Source: CAD feature listing. Evaluate the final solid. Frame: model axes, mm. A direction names the side the tool comes from. Coordinates: 2 decimals unless noted, no trailing zeros. Order: outer loops, then holes, each group sorted by start corner. A loop starts at its lowest first (then second) coordinate and runs counter-clockwise, first axis right, second up.
Autodesk Inventor part; units mm, degrees
ref_plane "YZ Plane" through (0, 0, 0) normal (1, 0, 0) x (0, 1, 0)
ref_plane "XZ Plane" through (0, 0, 0) normal (0, 1, 0) x (-1, 0, 0)
ref_plane "XY Plane" through (0, 0, 0) normal (0, 0, 1) x (1, 0, 0)
sketch "Sketch1" plane through (0, 0, 0) normal (0, 1, 0) x (-1, 0, 0)
  line L0 (-2.95, 2.95) -> (2.95, 2.95)
  line L1 (2.95, 2.95) -> (2.95, -2.95)
  line L2 (2.95, -2.95) -> (-2.95, -2.95)
  line L3 (-2.95, -2.95) -> (-2.95, 2.95)
  line L4 (-2.95, 2.95) -> (2.95, -2.95) construction
  line L5 (2.95, 2.95) -> (-2.95, -2.95) construction
  point P0 (0, 0)
  dimension "d0" = 5.9
  dimension "d1" = 5.9
extrude "Extrusion1" add sketch "Sketch1" along normal blind 16
sketch "Sketch2" plane through (0, 16, 0) normal (0, 1, 0) x (1, 0, 0)
  line L0 (4, -4) -> (-4, -4)
  line L1 (-4, -4) -> (-4, 4)
  line L2 (-4, 4) -> (4, 4)
  line L3 (4, 4) -> (4, -4)
  line L4 (4, -4) -> (-4, 4) construction
  line L5 (-4, -4) -> (4, 4) construction
  point P0 (0, 0)
  dimension "d4" = 8
  dimension "d5" = 8
extrude "Extrusion2" add sketch "Sketch2" along normal blind 60
chamfer "Chamfer1" distance 6 angle 45 1 edges at (0, 76, -4) measured on face at (1.3333, 76, 1.3333)
sketch "Sketch4" plane through (4, 76, 2) normal (0, 0.7071, -0.7071) x (-1, 0, 0)
  line L0 (8, -8.4853) -> (8, 0)
  line L1 (8, 0) -> (0, 0)
  line L2 (0, 0) -> (0, -8.4853)
  line L3 (0, -8.4853) -> (8, -8.4853)
  point P0 (4, -55.1543)
extrude "Extrusion4" add sketch "Sketch4" along normal blind 40
sketch "Sketch5" plane through (4, 104.2843, -26.2843) normal (0, 0.7071, -0.7071) x (-1, 0, 0)
  line L0 (8, -8.4853) -> (8, 0)
  line L1 (8, 0) -> (0, 0)
  line L2 (0, 0) -> (0, -8.4853)
  line L3 (0, -8.4853) -> (8, -8.4853)
  line L4 (7, -7.2426) -> (1, -7.2426)
  line L5 (1, -7.2426) -> (1, -1.2426)
  line L6 (1, -1.2426) -> (7, -1.2426)
  line L7 (7, -1.2426) -> (7, -7.2426)
  line L8 (7, -7.2426) -> (1, -1.2426) construction
  line L9 (1, -7.2426) -> (7, -1.2426) construction
  point P0 (4, -55.1543)
  point P1 (4, -4.2426)
  dimension "d15" = 6
  dimension "d16" = 6
extrude "Extrusion5" cut sketch "Sketch5" against normal blind 10 contours L4 L5 L6 L7
properties part number "Stalk"
Q1. Pull-direction query (X, two-part tool) for faces 1 (the flat face through (3, 98, -26)), 2 (the flat face through (0, 76, 3)), 3 (the flat face through (-3, 98, -26)), 4 (the flat face through (-4, 59, -3)); classes: pulls with the +X half, pulls with the -X half, needs draft (parallel to the pull), parting line crosses it, or undercut.
Solutions:
face 1: undercut
face 2: needs draft
face 3: undercut
face 4: pulls with the -X half
Q2. Section query C-C on y = 49.5. Output: boundary loops of the cut face in (x, z), plus the area to 3 significant figures.
Solutions:
outline: (-4, -4) - (4, -4) - (4, 4) - (-4, 4) - close
area: 64.0 mm2
Q3. Set-up query: faces 5 (the flat face through (-2.95, 8, 0)), 6 (the flat face through (-0.04, 95.68, -27.92)), 7 (the flat face through (0, 8, -2.95)). Return all of +Z, -Z, +X, -X, +Y, -Y with unobstructed straight access to the full face (end or side cutting, diameter ignored); none if empty.
Solutions:
face 5: +Z, -Z, -X, -Y
face 6: none
face 7: -Z, +X, -X, -Y
Q4. Material intervals for line 1 along Z through (x, y) = (2, 39); line 2 along Y through (x, z) = (-1, -27); line 3 along X through (y, z) = (97, -25), sorted ascending.
Solutions:
line 1: z = -4 to 4
line 2: y = 93 to 94.76, 103.24 to 103.57
line 3: x = -4 to -3, 3 to 4
Q5. Pin query (flat end, axial travel): P1, Ø2, axis at x = 0.5, y = 81.5, coming from the +Z side; P2, Ø6, axis at y = 86.5, z = -25, coming from the -X side; P3, Ø4.5, axis at y = 6, z = -0.5, coming from the +X side; P4, Ø1.6, axis at x = 1.5, z = 2.5, coming from the +Y side. Return the tip coordinate at first contact, or that it passes through.
Solutions:
P1: stops at z = -2.5
P2: passes through
P3: stops at x = 2.95
P4: stops at y = 76.3
Q6. Section query B-B on z = 1. Output: boundary loops of the cut face in (x, y), plus the area to 3 significant figures.
Solutions:
outline: (-4, 16) - (-2.95, 16) - (-2.95, 0) - (2.95, 0) - (2.95, 16) - (4, 16) - (4, 77) - (-4, 77) - close
area: 582 mm2
Q7. Section query D-D on z = -29. Output: boundary loops of the cut face in (x, y), plus the area to 3 significant figures.
Solutions:
outline: (-4, 95) - (4, 95) - (4, 101.57) - (3, 101.57) - (3, 96.76) - (-3, 96.76) - (-3, 101.57) - (-4, 101.57) - close
area: 23.7 mm2
